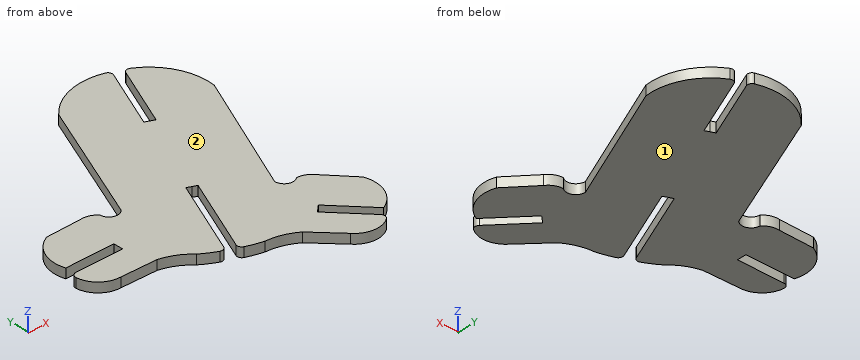
from build123d import *

# Parameters (mm, degrees)
BOSS_EXTRUDE1_DEPTH = 1.524


with BuildPart() as part:
    # Sketch1 → Boss-Extrude1 (new body)
    with BuildSketch(Plane.XY):
        with BuildLine():
            Line((-11.698031226, 1.301080189), (-17.241997575, 1.200259383))
            ThreePointArc((-17.241997575, 1.200259383), (-19.917117147, -1.466260827), (-20.124051829, -5.237702565))
            Line((-20.124051829, -5.237702565), (-12.408600231, -5.237702565))
            Line((-12.408600231, -5.237702565), (-12.408600231, -6.741954445))
            Line((-12.408600231, -6.741954445), (-19.871811516, -6.741954445))
            ThreePointArc((-19.871811516, -6.741954445), (-20.435206751, -6.990895181), (-20.630486437, -7.57506256))
            ThreePointArc((-20.630486437, -7.57506256), (-19.329359364, -10.115853363), (-16.636177401, -11.062067125))
            Line((-16.636177401, -11.062067125), (-10.972091682, -11.182579587))
            ThreePointArc((-10.972091682, -11.182579587), (-8.698171192, -12.023613454), (-6.754136813, -13.472331057))
            ThreePointArc((-6.754136813, -13.472331057), (-5.581948581, -14.227787409), (-4.346508881, -14.874647747))
            ThreePointArc((-4.346508881, -14.874647747), (-3.784346366, -14.895857379), (-3.377122413, -14.507726996))
            Line((-3.377122413, -14.507726996), (2.03023888, -2.061232355))
            Line((2.03023888, -2.061232355), (2.729092759, -2.364954689))
            Line((2.729092759, -2.364954689), (3.428024886, -2.668496912))
            Line((3.428024886, -2.668496912), (-1.97931368, -15.115001427))
            ThreePointArc((-1.97931368, -15.115001427), (-1.98510287, -15.677534117), (-1.585953772, -16.073963859))
            ThreePointArc((-1.585953772, -16.073963859), (-0.270018612, -16.535541807), (1.082127376, -16.876776006))
            ThreePointArc((1.082127376, -16.876776006), (3.467746446, -17.309065277), (5.634318126, -18.397191884))
            Line((5.634318126, -18.397191884), (9.587844362, -22.455026355))
            ThreePointArc((9.587844362, -22.455026355), (12.117419518, -23.777826074), (14.862522696, -22.994909661))
            ThreePointArc((14.862522696, -22.994909661), (15.156242938, -22.453509531), (14.953714903, -21.871815388))
            Line((14.953714903, -21.871815388), (9.860467214, -16.416693879))
            Line((9.860467214, -16.416693879), (10.959977394, -15.390121387))
            Line((10.959977394, -15.390121387), (16.22536578, -21.029614141))
            ThreePointArc((16.22536578, -21.029614141), (18.840822131, -18.304548485), (18.964246905, -14.529450993))
            Line((18.964246905, -14.529450993), (15.254476006, -10.408367691))
            ThreePointArc((15.254476006, -10.408367691), (14.298724728, -9.591322549), (13.07136856, -9.318155738))
            ThreePointArc((13.07136856, -9.318155738), (11.462041147, -9.532232913), (10.635341819, -8.134974174))
            Line((10.635341819, -8.134974174), (19.523278228, 11.967818074))
            ThreePointArc((19.523278228, 11.967818074), (18.552858543, 17.387639375), (14.725205948, 21.345574811))
            ThreePointArc((14.725205948, 21.345574811), (14.142053039, 21.397936165), (13.711309854, 21.001364186))
            Line((13.711309854, 21.001364186), (9.411697856, 11.104602687))
            Line((9.411697856, 11.104602687), (8.714639229, 11.412422878))
            Line((8.714639229, 11.412422878), (8.013937, 11.711856318))
            Line((8.013937, 11.711856318), (12.313567068, 21.608609967))
            ThreePointArc((12.313567068, 21.608609967), (12.30947588, 22.194094628), (11.873232067, 22.584607574))
            ThreePointArc((11.873232067, 22.584607574), (6.368068152, 22.681290418), (1.744271471, 19.691862119))
            Line((1.744271471, 19.691862119), (-6.884013371, -0.52373509))
            ThreePointArc((-6.884013371, -0.52373509), (-8.469497177, -0.873027031), (-9.411301698, 0.449382892))
            ThreePointArc((-9.411301698, 0.449382892), (-10.448574638, 1.160078409), (-11.698031226, 1.301080189))
        make_face()
    extrude(amount=BOSS_EXTRUDE1_DEPTH)


solid = part.part
The listing builds one solid part. Answer for the finished solid, in the listing's coordinates (mm). Face numbers are marked on the shaded views. Coordinates: 2 decimals unless noted, no trailing zeros. Write each loop counter-clockwise with the first axis right and the second up, starting at its lowest first coordinate (ties: lowest second). Pieces come first, ordered by that corner, then holes. Notation, with made-up numbers: (41.25, -4) - (96.25, -4) arc R16 ccw to (96.25, 10) - close; hole circle Ø1 at (20, 70). An arc over 180 degrees is marked (long way). Put each result on its own line as item: value.
1. The part is cut by section B-B on y = -4.5. Give the vertices of the cut face in (x, z).
Answer sheet:
outline: (-20.3, 0) - (0.97, 0) - (0.97, 1.52) - (-20.3, 1.52) - close; (2.63, 0) - (12.24, 0) - (12.24, 1.52) - (2.63, 1.52) - close
2. Flat-ended cylindrical pins translate along their axes: pin 1 Ø0.8 at (y, z) = (-6, 1) entering from -X; pin 2 Ø0.5 at (x, z) = (-16.5, 0.5) entering from -Y; pin 3 Ø0.5 at (x, z) = (-15.5, 0.5) entering from +Y. Find the tip coordinate at first contact, or state that the pin passes through.
Answer sheet:
pin 1: stops at x = -12.41
pin 2: stops at y = -11.07
pin 3: stops at y = 1.24
3. Determine the mould class of the marked faces 1 and 2 for opening direction Z: pulls with the +Z half, pulls with the -Z half, needs draft (parallel to the pull), parting line crosses it, or undercut.
Answer sheet:
face 1: pulls with the -Z half
face 2: pulls with the +Z half
4. The part is cut by section A-A on x = -0.5. Give the vertices of the cut face in (y, z).
Answer sheet:
outline: (-16.46, 0) - (-11.71, 0) - (-11.71, 1.52) - (-16.46, 1.52) - close; (-7.89, 0) - (14.43, 0) - (14.43, 1.52) - (-7.89, 1.52) - close
5. The part is cut by section C-C on y = 9. Give the vertices of the cut face in (x, z), plus the area to 3 significant figures.
Answer sheet:
outline: (-2.82, 0) - (18.21, 0) - (18.21, 1.52) - (-2.82, 1.52) - close
area: 32.1 mm^2
6. Find the intervals of material crossed by line 1 along Y through (x, z) = (12.5, 0.4); line 2 along Y through (x, z) = (-12.5, 1.4); line 3 along X through (y, z) = (-12, 0.5), in increasing order. Write a range as from..to.
Answer sheet:
line 1: y = -23.8..-19.24, -17.04..-9.63, -3.92..18.21
line 2: y = -11.15..-6.74, -5.24..1.29
line 3: x = -8.74..-2.29, -0.63..16.69
7. The part is cut by section D-D on y = 3.5. Give the vertices of the cut face in (x, z), plus the area to 3 significant figures.
Answer sheet:
outline: (-5.17, 0) - (15.78, 0) - (15.78, 1.52) - (-5.17, 1.52) - close
area: 31.9 mm^2
